Model file for the job. Use its own axes, mm. A direction names the side the tool comes from. Round coordinates to 2 decimals unless told otherwise and drop trailing zeros. Loops run counter-clockwise (first coordinate to the right, second up) from the corner with the lowest first, then second, coordinate; pieces in that order, holes last. Notation, with made-up numbers: M 69.5,23.25 L 73.5,23.25 A30 cw 73.5,58.25 Z; hole C 47,86 d7. An arc over 180 degrees is marked long. Use a Markdown table: item, result. Add a question column.
Item 1: Two-plate mould, pull along X, no slides. Class faces 4 (the flat face through (-40, 2, 39)), 5 (the cylindrical face through (0.88, 2.46, -39.99)), 6 (the flat face through (40, 2, 41)), 7 (the flat face through (-9, 5, 17)): +X half, -X half, draft (parallel to the pull), parting line (faces both ways), or undercut.
Item 2: Saw through at D-D on x = 14. Write the cut outline in (y, z).
Item 3: Pin check, flat tips, straight feed: P1, Ø4, axis at x = 15.5, y = 16, coming from the -Z side; P2, Ø2, axis at x = 23.5, z = -24, coming from the +Y side; P3, Ø10, axis at x = 26, z = 29, coming from the -Y side; P4, Ø5, axis at y = 16.5, z = 36.5, coming from the +X side. Stop position of each tip, or through.
Item 4: Wall check: L1, parallel to Y at x = 0, z = 60; L2, parallel to Z at x = 0, y = 2.8; L3, parallel to Y at x = 14.5, z = -27. Give the ranges that are in metal, low to high. Write a range as from..to.
Item 5: Saw through at B-B on z = -8. Write the cut outline in (x, y), then the cut area to 3 significant figures.
Item 6: Saw through at A-A on x = 0. Write the cut outline in (y, z), then the cut area to 4 significant figures.
Item 7: Saw through at C-C on z = 48.5. Write the cut outline in (x, y).
Item 8: Tool access for faces 1 (the cylindrical face through (-1.951, 5.214, 65.21)), 2 (the flat face through (-1, 0, 32)), 3 (the cylindrical face through (-0.88, 13.78, 39.99)): list every direction of +Z, -Z, +X, -X, +Y, -Y with a clear straight run to the whole face (end or side of a thin tool).
```python
from build123d import *

# Parameters (mm, degrees)
SKETCH1_R                                     = 19.05
PISTON_CONNECTION_PLATE_DEPTH                 = 5
SKETCH2_R                                     = 9
PLATFORM_TUBE_LINK_DEPTH                      = 80
ROD_START                                     = -50
SKETCH5_R                                     = 9
ROD_CAP_PREVENT_ROD_FROM_REACHING_PISTO_DEPTH = 50
CLEANUP_CUT_1_DEPTH                           = 94.722996111
CLEANUP_CUT_1_DEPTH_BACK                      = 94.722996111
SKETCH3_R                                     = 19.05
SKETCH4_R                                     = 40
CLEANUP_CUT_2_DEPTH                           = 93.352585349


with BuildPart() as part:
    # Sketch1 → Piston connection plate (new body)
    with BuildSketch(Plane(origin=(0, 0, 0), x_dir=(1, 0, 0), z_dir=(0, 1, 0))):
        with BuildLine():
            Line((-40, 0), (-40, -80))
            Line((-40, -80), (40, -80))
            Line((40, -80), (40, 0))
            ThreePointArc((40, 0), (0, 40), (-40, 0))
        make_face()
        with Locations(Location((0, 0, 0), (0, 0, 270))):
            Circle(SKETCH1_R, mode=Mode.SUBTRACT)
    extrude(amount=PISTON_CONNECTION_PLATE_DEPTH)

    # Sketch2 → Platform tube link (add)
    with BuildSketch(Plane.XY.offset(80)):
        with BuildLine():
            Line((-40, 5), (-7.552348551, 25.788215784))
            ThreePointArc((-7.552348551, 25.788215784), (0, 28), (7.552348551, 25.788215784))
            Line((7.552348551, 25.788215784), (40, 5))
            Line((40, 5), (40, 0))
            Line((40, 0), (-40, 0))
            Line((-40, 0), (-40, 5))
        make_face()
        with Locations((0, 14)):
            Circle(SKETCH2_R, mode=Mode.SUBTRACT)
    extrude(amount=-PLATFORM_TUBE_LINK_DEPTH)

    # Sketch5 → Rod cap (prevent rod from reaching piston) (add)
    with BuildSketch(Plane(origin=(0, 0, 0), x_dir=(-1, 0, 0), z_dir=(0, 0, -1)).offset(ROD_START)):
        with Locations(Location((0, 14, 0), (0, 0, 180))):
            Circle(SKETCH5_R)
    extrude(amount=ROD_CAP_PREVENT_ROD_FROM_REACHING_PISTO_DEPTH)

    # Sketch3 → Cleanup cut 1 (cut, two sides: drawn at the far end of the back side and taken through both)
    with BuildSketch(Plane.XZ.offset(-CLEANUP_CUT_1_DEPTH_BACK)):
        Circle(SKETCH3_R)
    extrude(amount=CLEANUP_CUT_1_DEPTH + CLEANUP_CUT_1_DEPTH_BACK, mode=Mode.SUBTRACT)

    # Sketch4 → Cleanup cut 2 (cut, through all)
    with BuildSketch(Plane(origin=(0, 5, 0), x_dir=(1, 0, 0), z_dir=(0, 1, 0))):
        Circle(SKETCH4_R)
    extrude(amount=CLEANUP_CUT_2_DEPTH, mode=Mode.SUBTRACT)


solid = part.part
```
Entries:
| question | item | result |
|---|---|---|
| 1 | face 4 | -X half |
| 1 | face 5 | parting line |
| 1 | face 6 | +X half |
| 1 | face 7 | undercut |
| 2 | outline | M 0,-37.47 L 5,-37.47 L 5,-12.92 L 0,-12.92 Z; M 0,12.92 L 5,12.92 L 5,37.47 L 21.66,37.47 L 21.66,80 L 0,80 Z |
| 3 | P1 | z = 35.97 |
| 3 | P2 | y = 5 |
| 3 | P3 | y = 0 |
| 3 | P4 | x = 25.95 |
| 4 | L1 | 0..5, 23..28 |
| 4 | L2 | -40..-19.05, 19.05..80 |
| 4 | L3 | 0..5 |
| 5 | outline | M -39.19,0 L -17.29,0 L -17.29,5 L -39.19,5 Z; M 17.29,0 L 39.19,0 L 39.19,5 L 17.29,5 Z |
| 5 | area | 219 mm2 |
| 6 | outline | M 0,-40 L 5,-40 L 5,-19.05 L 0,-19.05 Z; M 0,19.05 L 5,19.05 L 5,40 L 28,40 L 28,80 L 23,80 L 23,50 L 5,50 L 5,80 L 0,80 Z |
| 6 | area | 789.5 mm2 |
| 7 | outline | M -40,0 L 40,0 L 40,5 L 7.55,25.79 A14 ccw -7.55,25.79 L -40,5 Z |
| 8 | face 1 | +Z |
| 8 | face 2 | +Z, -Z, +X, -X, -Y |
| 8 | face 3 | -Z, +Y |
